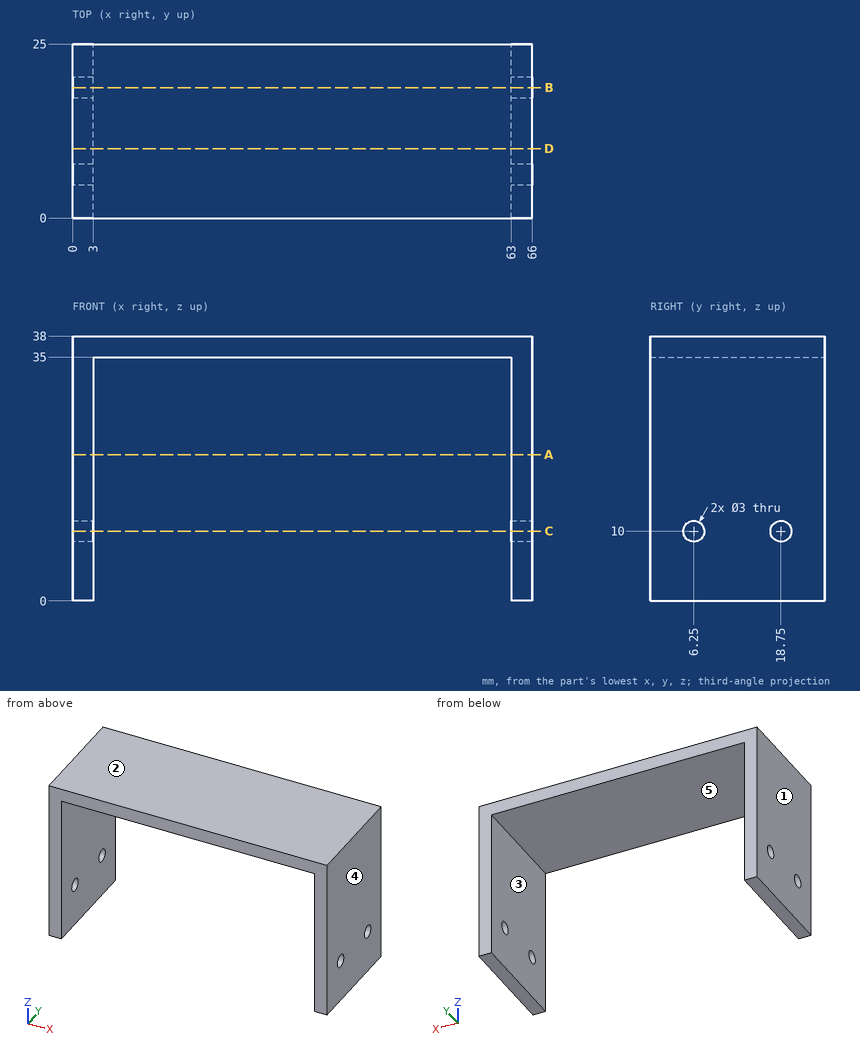
Print and shaded views of the part. All mm, measured from the part's lowest x, y and z. A direction names the side the tool comes from. Give positions to 0.01 mm unless a question says otherwise; leave off trailing zeros. Loops run counter-clockwise (first coordinate to the right, second up) from the corner with the lowest first, then second, coordinate; pieces in that order, holes last. Notation, with made-up numbers: (45, 65) -> (58, 65) arc R18 ccw to (58, 76) -> close; hole circle Ø3 at (-14.5, 5.5). An arc over 180 degrees is marked (long way). One line per question, with ' | ' between items. Start each with the question number.
1) Cut at B-B (y = 18.75). Give the cut face in (x, z), plus the area to 3 significant figures.
2) Cut at D-D (y = 10). Give the cut face in (x, z), plus the area to 3 significant figures.
3) Cut at C-C (z = 10). Give the cut face in (x, y).
4) Pin check, flat tips, straight feed: pin 1 (6 mm diameter, centred on y = 5.5, z = 9, fed in from -X); pin 2 (3 mm diameter, centred on x = 35.5, y = 4, fed in from -Z). Stop position of each tip, or through.
5) 3-axis set-ups, long thin cutter, end or side, ignore diameter. For the marked faces 4 and 5: which of +Z, -Z, +X, -X, +Y, -Y reach the whole face in a straight line?
6) Probe L1, parallel to X at y = 17, z = 32.5; L2, parallel to Z at x = 15.5, y = 15.25. List the from-to ranges inside material, lowest first.
7) Two-plate mould, pull along X, no slides. Class the marked faces 1, 2 and 3: released by +X, released by -X, zero draft, split by the parting line, or undercut.
8) Cut at A-A (z = 21). Give the cut face in (x, y), plus the area to 3 significant figures.
Return value:
1) outline: (0, 0) -> (3, 0) -> (3, 8.5) -> (0, 8.5) -> close; (0, 11.5) -> (3, 11.5) -> (3, 35) -> (63, 35) -> (63, 11.5) -> (66, 11.5) -> (66, 38) -> (0, 38) -> close; (63, 0) -> (66, 0) -> (66, 8.5) -> (63, 8.5) -> close | area: 390 mm^2
2) outline: (0, 0) -> (3, 0) -> (3, 35) -> (63, 35) -> (63, 0) -> (66, 0) -> (66, 38) -> (0, 38) -> close | area: 408 mm^2
3) outline: (0, 0) -> (3, 0) -> (3, 4.75) -> (0, 4.75) -> close; (0, 7.75) -> (3, 7.75) -> (3, 17.25) -> (0, 17.25) -> close; (0, 20.25) -> (3, 20.25) -> (3, 25) -> (0, 25) -> close; (63, 0) -> (66, 0) -> (66, 4.75) -> (63, 4.75) -> close; (63, 7.75) -> (66, 7.75) -> (66, 17.25) -> (63, 17.25) -> close; (63, 20.25) -> (66, 20.25) -> (66, 25) -> (63, 25) -> close
4) pin 1: x = 0 | pin 2: z = 35
5) face 4: +Z, -Z, +X, +Y, -Y | face 5: -Z, +Y, -Y
6) L1: 0 to 3, 63 to 66 | L2: 35 to 38
7) face 1: released by -X | face 2: zero draft | face 3: undercut
8) outline: (0, 0) -> (3, 0) -> (3, 25) -> (0, 25) -> close; (63, 0) -> (66, 0) -> (66, 25) -> (63, 25) -> close | area: 150 mm^2
